from build123d import *


with BuildPart() as part:
    # Schizzo1 → Rivoluzione1 (revolve)
    with BuildSketch(Plane.XY, mode=Mode.PRIVATE) as rivoluzione1_sk:
        with BuildLine():
            Line((0, 64.35), (1, 63.35))
            Line((1, 63.35), (4.561250083, 63.35))
            ThreePointArc((4.561250083, 63.35), (9.32995439, 68.154290191), (16.039607805, 69.05))
            Line((16.039607805, 69.05), (27.333333333, 69.05))
            ThreePointArc((27.333333333, 69.05), (27.804737854, 69.245262146), (28, 69.716666667))
            Line((28, 69.716666667), (28, 74))
            ThreePointArc((28, 74), (27.707106781, 74.707106781), (27, 75))
            Line((27, 75), (2, 75))
            ThreePointArc((2, 75), (0.585786438, 74.414213562), (0, 73))
            Line((0, 73), (0, 64.35))
        make_face()
    revolve(rivoluzione1_sk.sketch.rotate(Axis((28, 0, 0), (-1, 0, 0)), 270), axis=Axis((28, 0, 0), (-1, 0, 0)))


solid = part.part
The model under review builds one solid part; all positions refer to its coordinate system, in mm. Round coordinates to 2 decimals unless told otherwise and drop trailing zeros. Order: outer loops, then holes, each group sorted by start corner. A loop starts at its lowest first (then second) coordinate and runs counter-clockwise, first axis right, second up. Notation, with made-up numbers: (-21, 30) -> (17, 30) arc R11 cw to (17, 41) -> close; hole circle Ø7 at (78, 74). An arc over 180 degrees is marked (long way). Write item = value, one per line. Start each with the question number.
Item 1: Consider section A-A on z = 0. Write out the cut boundary in (x, y).
Item 2: Consider section C-C on x = 13.5. Write out the cut boundary in (y, z), plus the area to 3 significant figures.
Item 3: For line 1 along Y through (x, z) = (2.8, 0); line 2 along Z through (x, y) = (13.5, 43.5); line 3 along Y through (x, z) = (23.75, 0), list the stretches that pass through material, from the lowest coordinate up.
Item 4: Clearance check with flat-ended pins moving along their axes: pin 1 Ø8 at (x, y) = (4.5, -49.5) entering from -Z; pin 2 Ø8 at (x, y) = (23.5, 32) entering from -Z; pin 3 Ø10 at (x, y) = (7.5, 36) entering from +Z. State where each tip first meets the part, or that it passes through.
Item 5: Mouldability with a two-part tool opening along Z and no side actions: class faces 1 (the face through (2.806, -61.844, -13.733)), 2 (the face through (28, 50, 50)), 3 (the face through (14.325, -45.636, -59.517)), 4 (the face through (21.8, -67.4, -15)) as released by +Z, released by -Z, zero draft, split by the parting line, or undercut.
Conclusion:
q1.outline = (0, -73) arc R2 ccw to (2, -75) -> (27, -75) arc R1 ccw to (28, -74) -> (28, -69.72) arc R0.67 ccw to (27.33, -69.05) -> (16.04, -69.05) arc R10.5 cw to (4.56, -63.35) -> (1, -63.35) -> (0, -64.35) -> close; (0, 64.35) -> (1, 63.35) -> (4.56, 63.35) arc R10.5 cw to (16.04, 69.05) -> (27.33, 69.05) arc R0.67 ccw to (28, 69.72) -> (28, 74) arc R1 ccw to (27, 75) -> (2, 75) arc R2 ccw to (0, 73) -> close
q2.outline = circle Ø150 at (0, 0); hole circle Ø138.48 at (0, 0)
q2.area = 2,610 mm2
q3.line_1 = -75 to -63.35, 63.35 to 75
q3.line_2 = -61.1 to -53.87, 53.87 to 61.1
q3.line_3 = -75 to -69.05, 69.05 to 75
q4.pin_1 = -59.62
q4.pin_2 = -69.58
q4.pin_3 = 68.29
q5.face_1 = undercut
q5.face_2 = zero draft
q5.face_3 = split by the parting line
q5.face_4 = undercut
